```python
from build123d import *

# Parameters (mm, degrees)
SKETCH_1_R          = 1.5
EXTRUDE_1_DEPTH     = 5
SKETCH_2_R          = 1.5
CUT_EXTRUDE_4_DEPTH = 9


with BuildPart() as part:
    # Эскиз1 → Бобышка-Вытянуть1 (new body)
    with BuildSketch(Plane(origin=(0, 0, 0), x_dir=(1, 0, 0), z_dir=(0, 1, 0))):
        with BuildLine():
            Line((0, 10), (0, 2))
            ThreePointArc((0, 2), (0.765366865, 1.847759065), (1.414213562, 1.414213562))
            Line((1.414213562, 1.414213562), (3.556747109, 3.556747109))
            ThreePointArc((3.556747109, 3.556747109), (3.556747109, 5.678067453), (5.678067453, 5.678067453))
            Line((5.678067453, 5.678067453), (7.071067812, 7.071067812))
            ThreePointArc((7.071067812, 7.071067812), (3.826834324, 9.238795325), (0, 10))
        make_face()
        with BuildLine():
            ThreePointArc((2, 0), (-1.414213562, -1.414213562), (0, 2))
            Line((0, 2), (0, 10))
            ThreePointArc((0, 10), (-7.071067812, -7.071067812), (10, 0))
            ThreePointArc((10, 0), (9.238795325, 3.826834324), (7.071067812, 7.071067812))
            Line((7.071067812, 7.071067812), (5.678067453, 5.678067453))
            ThreePointArc((5.678067453, 5.678067453), (6.00322658, 5.19143243), (6.117407281, 4.617407281))
            ThreePointArc((6.117407281, 4.617407281), (5.19143243, 3.231587982), (3.556747109, 3.556747109))
            Line((3.556747109, 3.556747109), (1.414213562, 1.414213562))
            ThreePointArc((1.414213562, 1.414213562), (1.847759065, 0.765366865), (2, 0))
        make_face()
        with Locations((-4.617407281, -4.617407281)):
            Circle(SKETCH_1_R, mode=Mode.SUBTRACT)
        with Locations((4.617407281, -4.617407281)):
            Circle(SKETCH_1_R, mode=Mode.SUBTRACT)
        with Locations((-4.617407281, 4.617407281)):
            Circle(SKETCH_1_R, mode=Mode.SUBTRACT)
    extrude(amount=EXTRUDE_1_DEPTH)

    # Эскиз2 → Вырез-Вытянуть4 (cut)
    with BuildSketch(Plane(origin=(10, 0, 0), x_dir=(0, 0, -1), z_dir=(1, 0, 0))):
        with Locations((0, 2.5)):
            Circle(SKETCH_2_R)
    extrude(amount=-CUT_EXTRUDE_4_DEPTH, mode=Mode.SUBTRACT)


solid = part.part
```
Can you work these out from the model? Positions are in its coordinate system, mm. A direction names the side the tool comes from. Give positions to 0.01 mm unless a question says otherwise; leave off trailing zeros. Write each loop counter-clockwise with the first axis right and the second up, starting at its lowest first coordinate (ties: lowest second). Pieces come first, ordered by that corner, then holes. Notation, with made-up numbers: (-4, -7.5) -> (11, -7.5) arc R17 cw to (11, 5.5) -> close; hole circle Ø9 at (1, 72). An arc over 180 degrees is marked (long way). One line per item, written item: value.
Q1. We'd pull the mould along X, two halves only. Please class faces 3 (the face through (-5.81, 2.46, 5.53)), 4 (the face through (-2.4, 5, -0.1)): +X half, -X half, draft (parallel to the pull), parting line (faces both ways), or undercut.
Results found:
face 3: undercut
face 4: draft
Q2. Imagine slicing it at D-D on z = 5. Please give me the cut outline in (x, y).
Results found:
outline: (-8.66, 0) -> (-6.07, 0) -> (-6.07, 5) -> (-8.66, 5) -> close; (-3.17, 0) -> (3.17, 0) -> (3.17, 5) -> (-3.17, 5) -> close; (6.07, 0) -> (8.66, 0) -> (8.66, 5) -> (6.07, 5) -> close
Q3. Imagine slicing it at A-A on z = -1. Please give me the cut outline in (x, y), and give its area (3 significant figures).
Results found:
outline: (-9.95, 0) -> (-1.73, 0) -> (-1.73, 5) -> (-9.95, 5) -> close; (1.73, 0) -> (9.95, 0) -> (9.95, 1.38) -> (1.73, 1.38) -> close; (1.73, 3.62) -> (9.95, 3.62) -> (9.95, 5) -> (1.73, 5) -> close
area: 63.8 mm^2
Q4. For P1, Ø1.5, axis at x = 2.5, y = 1, coming from the +Z side; P2, Ø1, axis at y = 2, z = 5, coming from the -X side; P3, Ø1.5, axis at x = -6, y = 2.5, coming from the -Z side; P4, Ø2.5, axis at x = 0, z = 0, coming from the -Y side, each with a flat end and sliding along its axis, tell me the tip position at first contact or that it passes through.
Results found:
P1: stops at z = 9.85
P2: stops at x = -8.93
P3: stops at z = -8.51
P4: passes through
Q5. Imagine slicing it at B-B on y = 0.75. Please give me the cut outline in (x, z).
Results found:
outline: circle Ø20 at (0, 0); hole circle Ø3 at (-4.62, -4.62); hole circle Ø3 at (-4.62, 4.62); hole circle Ø4 at (0, 0); hole circle Ø3 at (4.62, -4.62); hole circle Ø3 at (4.62, 4.62)
Q6. Please list where these lines run through material, in increasing order: line 1 (Z direction, x = 0, y = 2.05); line 2 (Z direction, x = 4.25, y = 2); line 3 (Z direction, x = -5.25, y = 4.35). Write a range as [from, to].
Results found:
line 1: z = [-10, -2], [2, 10]
line 2: z = [-9.05, -6.07], [-3.16, -1.41], [1.41, 3.16], [6.07, 9.05]
line 3: z = [-8.51, -5.98], [-3.26, 3.26], [5.98, 8.51]
Q7. Imagine slicing it at C-C on y = 2.5. Please give me the cut outline in (x, z).
Results found:
outline: (1.32, -1.5) arc R2 cw (long way) to (1.32, 1.5) -> (9.89, 1.5) arc R10 ccw (long way) to (9.89, -1.5) -> close; hole circle Ø3 at (-4.62, -4.62); hole circle Ø3 at (-4.62, 4.62); hole circle Ø3 at (4.62, -4.62); hole circle Ø3 at (4.62, 4.62)
Q8. Which directions (+Z, -Z, +X, -X, +Y, -Y) give clear straight access to the entire face, cutting with the end or side of a thin tool? Please do faces 1 (the face through (6, 4, 0)), 2 (the face through (6, 2.5, 5.2)).
Results found:
face 1: +X
face 2: +Y, -Y
